Design review of the part built by this model. Coordinates are the model's own, in mm. A direction names the side the tool comes from. Coordinates: 2 decimals unless noted, no trailing zeros. Loops run counter-clockwise (first coordinate to the right, second up) from the corner with the lowest first, then second, coordinate; pieces in that order, holes last. Notation, with made-up numbers: (83.5, 8) - (137.5, 8) arc R31 ccw to (137.5, 47) - close; hole circle Ø2 at (52, 74). An arc over 180 degrees is marked (long way). Answer in a Markdown table with one row per item. Add a question column.
(1) Clearance check with a flat-ended pin moving along its axis: pin 1 (2 mm diameter, centred on x = -69.5, z = 2.5, fed in from -Y). State where the tip first meets the part, or that it passes through.
(2) The part is to be moulded in two halves that separate along X. For faces 1 (the face through (-93, -15.714, 4)), 2 (the face through (-96.583, -9, 4)), 3 (the face through (62.795, -4.13, 3.519)), 4 (the face through (-15, -5.314, 4)), say which applies: released by +X, released by -X, zero draft, split by the parting line, or undercut.
(3) For faces 5 (the face through (-91.057, -4.13, 3.519)), 6 (the face through (-94.11, -14.5, 3.52)), 7 (the face through (65.269, -9, 4)), list the 3-axis set-ups (+Z, -Z, +X, -X, +Y, -Y) from which the entire face can be reached by the end or side of a thin tool; tool diameter is ignored.
(4) To check wall thickness, follow L1, parallel to X at y = -3.5, z = 4.25; L2, parallel to Y at x = 9.5, z = 5.25; L3, parallel to X at y = -4.25, z = 2.75. State the ranges of each line that lie inside material, in increasing order. Write a range as [from, to].
(5) We need section A-A, the plane x = -69. Write out the cut boundary in (y, z), plus the area to 3 significant figures.
from build123d import *

# Parameters (mm, degrees)
SKETCH_1_W      = 4
SKETCH_1_H      = 8
SKETCH_1_W_2    = 153.851648
EXTRUDE_1_DEPTH = 8
SKETCH_2_R      = 1.6
EXTRUDE_2_DEPTH = 2.4
SKETCH_3_R      = 1.6
SKETCH_3_R_2    = 1.65
EXTRUDE_3_DEPTH = 2.4


with BuildPart() as part:
    # 草图1 → 凸台-拉伸1 (new body)
    with BuildSketch(Plane.XY):
        with Locations((-94.582983627, -9.313586075)):
            Rectangle(SKETCH_1_W, SKETCH_1_H)
        with Locations((-15.657159627, -9.313586075)):
            Rectangle(SKETCH_1_W_2, SKETCH_1_H)
        with Locations((63.268664373, -9.313586075)):
            Rectangle(SKETCH_1_W, SKETCH_1_H)
    extrude(amount=EXTRUDE_1_DEPTH)

    # 草图2 → 凸台-拉伸2 (add)
    with BuildSketch(Plane(origin=(0, -5.313586075, 0), x_dir=(1, 0, 0), z_dir=(0, 1, 0))):
        with Locations((-92.582983627, -4)):
            Circle(SKETCH_2_R)
        with Locations((61.268664373, -4)):
            Circle(SKETCH_2_R)
    extrude(amount=EXTRUDE_2_DEPTH)

    # 草图3 → 凸台-拉伸3 (add)
    with BuildSketch(Plane(origin=(0, -13.313586075, 0), x_dir=(-1, 0, 0), z_dir=(0, -1, 0))):
        with Locations((92.582983627, -4)):
            Circle(SKETCH_3_R)
        with Locations((-61.268664373, -4)):
            Circle(SKETCH_3_R_2)
    extrude(amount=EXTRUDE_3_DEPTH)


solid = part.part
Responses:
| question | item | result |
|---|---|---|
| 1 | pin 1 | stops at y = -13.31 |
| 2 | face 1 | zero draft |
| 2 | face 2 | released by -X |
| 2 | face 3 | undercut |
| 2 | face 4 | undercut |
| 3 | face 5 | +Y |
| 3 | face 6 | -Y |
| 3 | face 7 | +Z, -Z, +X, +Y, -Y |
| 4 | L1 | x = [-94.16, -91], [59.69, 62.85] |
| 4 | L2 | y = [-13.31, -5.31] |
| 4 | L3 | x = [-93.58, -91.58], [60.27, 62.27] |
| 5 | outline | (-13.31, 0) - (-5.31, 0) - (-5.31, 8) - (-13.31, 8) - close |
| 5 | area | 64.0 mm2 |
